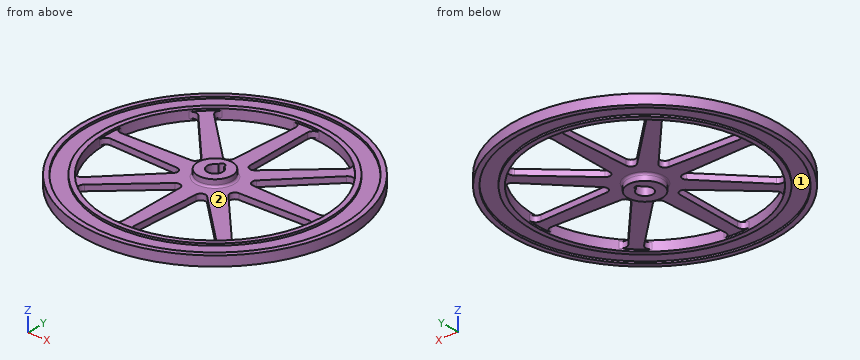
from build123d import *

# Parameters (mm, degrees)
SKETCH1_R           = 17.5
BOSS_EXTRUDE1_DEPTH = 10
SKETCH1_4_R         = 130
SKETCH1_4_R_2       = 115
SKETCH1_4_R_3       = 17.5
BOSS_EXTRUDE3_DEPTH = 3
SKETCH1_5_R         = 135
SKETCH1_5_R_2       = 130
SKETCH1_5_R_3       = 115
SKETCH1_5_R_4       = 110
BOSS_EXTRUDE4_DEPTH = 5
FILLET1_R           = 6
FILLET2_R           = 2


with BuildPart() as part:
    # Sketch1 → Boss-Extrude1 (new, symmetric)
    with BuildSketch(Plane.XY):
        Circle(SKETCH1_R)
        with BuildLine():
            ThreePointArc((2.946793809, 7.4375), (6.617187865, 4.495867521), (8, 0))
            ThreePointArc((8, 0), (-4.495867521, -6.617187865), (-2.946793809, 7.4375))
            ThreePointArc((-2.946793809, 7.4375), (0, 11), (2.946793809, 7.4375))
        make_face(mode=Mode.SUBTRACT)
    extrude(amount=BOSS_EXTRUDE1_DEPTH, both=True)

    # Sketch1_4 → Boss-Extrude3 (add, symmetric)
    # profile 1 of 2: a face of its own
    with BuildSketch(Plane.XY):
        Circle(SKETCH1_4_R)
        Circle(SKETCH1_4_R_2, mode=Mode.SUBTRACT)
    # profile 2 of 2: a face of its own
    with BuildSketch(Plane.XY):
        with BuildLine():
            Line((8.396299036, 32.18156505), (6, 109.836241742))
            ThreePointArc((6, 109.836241742), (0, 110), (-6, 109.836241742))
            Line((-6, 109.836241742), (-8.396299036, 32.18156505))
            ThreePointArc((-8.396299036, 32.18156505), (-11.480502971, 27.716385975), (-16.818722891, 28.692882861))
            Line((-16.818722891, 28.692882861), (-73.423310669, 81.908592043))
            ThreePointArc((-73.423310669, 81.908592043), (-77.781745931, 77.781745931), (-81.908592043, 73.423310669))
            Line((-81.908592043, 73.423310669), (-28.692882861, 16.818722891))
            ThreePointArc((-28.692882861, 16.818722891), (-27.716385975, 11.480502971), (-32.18156505, 8.396299036))
            Line((-32.18156505, 8.396299036), (-109.836241742, 6))
            ThreePointArc((-109.836241742, 6), (-110, 0), (-109.836241742, -6))
            Line((-109.836241742, -6), (-32.18156505, -8.396299036))
            ThreePointArc((-32.18156505, -8.396299036), (-27.716385975, -11.480502971), (-28.692882861, -16.818722891))
            Line((-28.692882861, -16.818722891), (-81.908592043, -73.423310669))
            ThreePointArc((-81.908592043, -73.423310669), (-77.781745931, -77.781745931), (-73.423310669, -81.908592043))
            Line((-73.423310669, -81.908592043), (-16.818722891, -28.692882861))
            ThreePointArc((-16.818722891, -28.692882861), (-11.480502971, -27.716385975), (-8.396299036, -32.18156505))
            Line((-8.396299036, -32.18156505), (-6, -109.836241742))
            ThreePointArc((-6, -109.836241742), (0, -110), (6, -109.836241742))
            Line((6, -109.836241742), (8.396299036, -32.18156505))
            ThreePointArc((8.396299036, -32.18156505), (11.480502971, -27.716385975), (16.818722891, -28.692882861))
            Line((16.818722891, -28.692882861), (73.423310669, -81.908592043))
            ThreePointArc((73.423310669, -81.908592043), (77.781745931, -77.781745931), (81.908592043, -73.423310669))
            Line((81.908592043, -73.423310669), (28.692882861, -16.818722891))
            ThreePointArc((28.692882861, -16.818722891), (27.716385975, -11.480502971), (32.18156505, -8.396299036))
            Line((32.18156505, -8.396299036), (109.836241742, -6))
            ThreePointArc((109.836241742, -6), (109.959052814, -3.001117157), (110, 0))
            ThreePointArc((110, 0), (109.959052814, 3.001117157), (109.836241742, 6))
            Line((109.836241742, 6), (32.18156505, 8.396299036))
            ThreePointArc((32.18156505, 8.396299036), (27.716385975, 11.480502971), (28.692882861, 16.818722891))
            Line((28.692882861, 16.818722891), (81.908592043, 73.423310669))
            ThreePointArc((81.908592043, 73.423310669), (77.781745931, 77.781745931), (73.423310669, 81.908592043))
            Line((73.423310669, 81.908592043), (16.818722891, 28.692882861))
            ThreePointArc((16.818722891, 28.692882861), (11.480502971, 27.716385975), (8.396299036, 32.18156505))
        make_face()
        Circle(SKETCH1_4_R_3, mode=Mode.SUBTRACT)
    extrude(amount=BOSS_EXTRUDE3_DEPTH, both=True)


with BuildPart() as boss_extrude3_piece_1:
    # of the separate pieces the step leaves, piece 1, a body of its own (boss_extrude3_pieces)
    add(part.part.solids().sort_by_distance((17.5, 0, -10))[0])



with BuildPart() as boss_extrude3_piece_2:
    # of the separate pieces the step leaves, piece 2, a body of its own (boss_extrude3_pieces)
    add(part.part.solids().sort_by_distance((130, 0, -3))[0])


with BuildPart() as boss_extrude3_piece_1_1:
    add(boss_extrude3_piece_1.part)

    add(boss_extrude3_piece_2.part)  # Boss-Extrude4 merges Boss-Extrude3 piece 2
    # Sketch1_5 → Boss-Extrude4 (add, symmetric)
    # profile 1 of 2: a face of its own
    with BuildSketch(Plane.XY):
        Circle(SKETCH1_5_R)
        Circle(SKETCH1_5_R_2, mode=Mode.SUBTRACT)
    # profile 2 of 2: a face of its own
    with BuildSketch(Plane.XY):
        Circle(SKETCH1_5_R_3)
        Circle(SKETCH1_5_R_4, mode=Mode.SUBTRACT)
    extrude(amount=BOSS_EXTRUDE4_DEPTH, both=True)

    # Fillet1
    fillet1_edges = [boss_extrude3_piece_1_1.edges().sort_by_distance(p)[0] for p in [
        (-109.836241742, 6, 0),
        (-109.836241742, -6, 0),
        (-81.908592043, -73.423310669, 0),
        (-73.423310669, -81.908592043, 0),
        (-6, -109.836241742, 0),
        (6, -109.836241742, 0),
        (73.423310669, -81.908592043, 0),
        (81.908592043, -73.423310669, 0),
        (109.836241742, -6, 0),
        (109.836241742, 6, 0),
        (81.908592043, 73.423310669, 0),
        (73.423310669, 81.908592043, 0),
        (6, 109.836241742, 0),
        (-6, 109.836241742, 0),
        (-73.423310669, 81.908592043, 0),
        (-81.908592043, 73.423310669, 0),
    ]]
    fillet(fillet1_edges, radius=FILLET1_R)

    # Fillet2
    fillet2_edges = [boss_extrude3_piece_1_1.edges().sort_by_distance(p)[0] for p in [
        (-17.5, 0, -3),
        (-17.5, 0, 3),
    ]]
    fillet(fillet2_edges, radius=FILLET2_R)


solid = boss_extrude3_piece_1_1.part
CAD build for the part. Positions are in the model's coordinates, mm. Face numbers are marked on the shaded views. A direction names the side the tool comes from. Coordinates: 2 decimals unless noted, no trailing zeros. Answer as a JSON object with one key per item and string values. Group by question number.
1) Wall check: line 1 (Y direction, x = 0, z = 1.5); line 2 (Y direction, x = 60, z = 0.5); line 3 (X direction, y = -41.5, z = 2.5). Give the ranges that are in metal, low to high. Write a range as from..to.
2) Pin check, flat tips, straight feed: pin 1 Ø2 at (y, z) = (17, -0.5) entering from -X; pin 2 Ø8 at (x, z) = (30.5, -6.5) entering from +Y; pin 3 Ø8 at (x, y) = (-95, 95.5) entering from +Z; pin 4 Ø3.5 at (x, y) = (0, 8) entering from +Z. Stop position of each tip, or through.
3) Saw through at A-A (y = 38). Give the number of separate pieces and of enclosed holes in the cut face, plus the area to 3 significant figures.
4) Tool access for the marked faces 1 and 2: list every direction of +Z, -Z, +X, -X, +Y, -Y with a clear straight run to the whole face (end or side of a thin tool).
Values follow:
{
 "1": {"line 1": "y = -135..-8, 11..135", "line 2": "y = -120.93..-92.2, -69.29..-50.12, -7.54..7.54, 50.12..69.29, 92.2..120.93", "line 3": "x = -128.46..-101.87, -51.9..-30.44, -8.11..8.11, 30.44..51.9, 101.87..128.46"},
 "2": {"pin 1": "stops at x = -134.05", "pin 2": "stops at y = 132.31", "pin 3": "stops at z = 5", "pin 4": "passes through"},
 "3": {"separate pieces": "5", "enclosed holes": "0", "area": "761 mm2"},
 "4": {"face 1": "-Z", "face 2": "+Z"}
}
